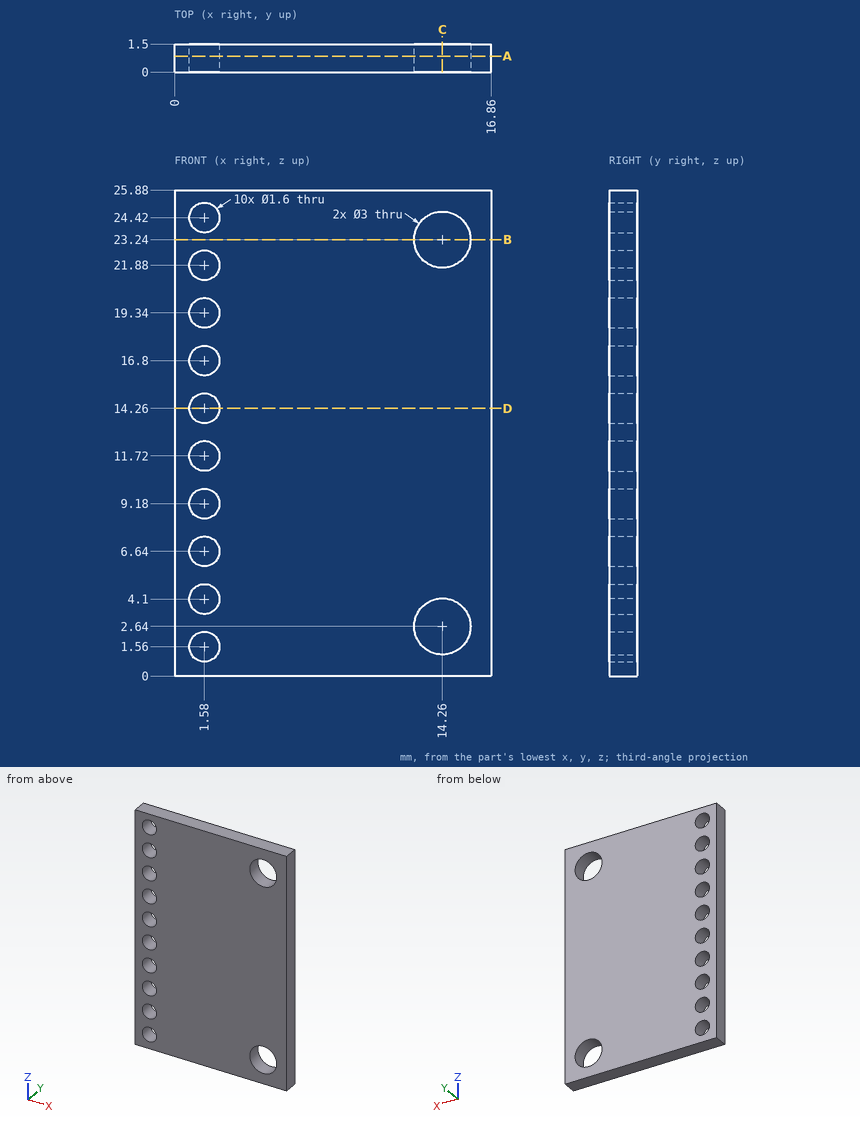
For this review, use the dimensioned drawing (mm, ordinates from the lowest corner) and the shaded views. Round coordinates to 2 decimals unless told otherwise and drop trailing zeros. Loops run counter-clockwise (first coordinate to the right, second up) from the corner with the lowest first, then second, coordinate; pieces in that order, holes last. Notation, with made-up numbers: (41.25, -28.5) -> (90.25, -28.5) arc R26 cw to (90.25, -5.5) -> close; hole circle Ø3 at (47.5, -12). An arc over 180 degrees is marked (long way). Write item = value, one per line. Start each with the question number.
Item 1: Take a section at C-C on x = 14.26. Give the boundary of the cut face in (y, z), plus the area to 3 significant figures.
Item 2: Take a section at A-A on y = 0.85. Count the separate pieces of the cut face and the enclosed holes in it, plus the area to 3 significant figures.
Item 3: To check wall thickness, follow L1, parallel to Z at x = 14.26, y = 0.6; L2, parallel to X at y = 0.5, z = 16.8; L3, parallel to X at y = 0.5, z = 23.24. State the ranges of each line that lie inside material, in increasing order.
Item 4: Insertion check: pin 1 (1.4 mm diameter, centred on x = 1.58, z = 14.26, fed in from -Y). The pin has a flat end and moves straight along its axis. Give the tip position at first contact, or say it passes through.
Item 5: Take a section at B-B on z = 23.24. Give the boundary of the cut face in (x, y), plus the area to 3 significant figures.
Item 6: Take a section at D-D on z = 14.26. Give the boundary of the cut face in (x, y), plus the area to 3 significant figures.
Result:
q1.outline = (0, 0) -> (1.5, 0) -> (1.5, 1.14) -> (0, 1.14) -> close; (0, 4.14) -> (1.5, 4.14) -> (1.5, 21.74) -> (0, 21.74) -> close; (0, 24.74) -> (1.5, 24.74) -> (1.5, 25.88) -> (0, 25.88) -> close
q1.area = 29.8 mm²
q2.separate_pieces = 1
q2.enclosed_holes = 12
q2.area = 402 mm²
q3.L1 = 0 to 1.14, 4.14 to 21.74, 24.74 to 25.88
q3.L2 = 0 to 0.78, 2.38 to 16.86
q3.L3 = 0 to 12.76, 15.76 to 16.86
q4.pin_1 = through
q5.outline = (0, 0) -> (12.76, 0) -> (12.76, 1.5) -> (0, 1.5) -> close; (15.76, 0) -> (16.86, 0) -> (16.86, 1.5) -> (15.76, 1.5) -> close
q5.area = 20.8 mm²
q6.outline = (0, 0) -> (0.78, 0) -> (0.78, 1.5) -> (0, 1.5) -> close; (2.38, 0) -> (16.86, 0) -> (16.86, 1.5) -> (2.38, 1.5) -> close
q6.area = 22.9 mm²
